```python
from build123d import *

# Parameters (mm, degrees)
BOSS_EXTRUDE1_DEPTH      = 3
BOSS_EXTRUDE1_DEPTH_BACK = 3
FILLET1_R                = 5


with BuildPart() as part:
    # Sketch1 → Boss-Extrude1 (new, two sides: drawn at the far end of the back side and taken through both)
    with BuildSketch(Plane(origin=(0, 0, 0), x_dir=(1, 0, 0), z_dir=(0, 1, 0)).offset(-BOSS_EXTRUDE1_DEPTH_BACK)):
        with BuildLine():
            Line((16.248076809, -15.5), (32.5, -15.5))
            Line((32.5, -15.5), (32.5, 15.5))
            Line((32.5, 15.5), (-32.5, 15.5))
            Line((-32.5, 15.5), (-32.5, -15.5))
            Line((-32.5, -15.5), (-16.248076809, -15.5))
            ThreePointArc((-16.248076809, -15.5), (0, 6.5), (16.248076809, -15.5))
        make_face()
    extrude(amount=BOSS_EXTRUDE1_DEPTH + BOSS_EXTRUDE1_DEPTH_BACK)

    # Fillet1
    fillet1_edges = [part.edges().sort_by_distance(p)[0] for p in [
        (16.248076809, 0, 15.5),
        (-16.248076809, 0, 15.5),
    ]]
    fillet(fillet1_edges, radius=FILLET1_R)


solid = part.part
```
Part model, mm, in its own coordinate system. A direction names the side the tool comes from. Round coordinates to 2 decimals unless told otherwise and drop trailing zeros. Write each loop counter-clockwise with the first axis right and the second up, starting at its lowest first coordinate (ties: lowest second). Pieces come first, ordered by that corner, then holes.
Item 1: Probe L1, parallel to X at y = -2.7, z = 1; L2, parallel to X at y = 1.6, z = -0.5; L3, parallel to Z at x = 4, y = 2.3. List the from-to ranges inside material, lowest first.
Results:
L1: x = -32.5 to -14.1, 14.1 to 32.5
L2: x = -32.5 to -12.96, 12.96 to 32.5
L3: z = -15.5 to -6.02
Item 2: Which spindle directions (+Z, -Z, +X, -X, +Y, -Y) get a long thin tool onto all of the face, cutting with end or side? Do faces 1 (the flat face through (0, 0, -15.5)), 2 (the cylindrical face through (-18.5, 0.04, 14.07)). Say none if no direction does.
Results:
face 1: -Z, +X, -X, +Y, -Y
face 2: +Z, +Y, -Y
Item 3: Cut at A-A, the plane z = 6. Give the cut face in (x, y).
Results:
outline: (-32.5, -3) - (-16.39, -3) - (-16.39, 3) - (-32.5, 3) - close; (16.39, -3) - (32.5, -3) - (32.5, 3) - (16.39, 3) - close
Item 4: Cut at C-C, the plane x = 0. Give the cut face in (y, z), plus the area to 3 significant figures.
Results:
outline: (-3, -15.5) - (3, -15.5) - (3, -6.5) - (-3, -6.5) - close
area: 54.0 mm2
Item 5: Cut at B-B, the plane y = 1. Give the cut face in (x, z).
Results:
outline: (-32.5, -15.5) - (32.5, -15.5) - (32.5, 15.5) - (22, 15.5) arc R5 ccw to (17, 10.5) arc R17 cw to (-17, 10.5) arc R5 ccw to (-22, 15.5) - (-32.5, 15.5) - close
Item 6: Cut at D-D, the plane z = -2. Give the cut face in (x, y), plus the area to 3 significant figures.
Results:
outline: (-32.5, -3) - (-11.52, -3) - (-11.52, 3) - (-32.5, 3) - close; (11.52, -3) - (32.5, -3) - (32.5, 3) - (11.52, 3) - close
area: 252 mm2
